Design review of the part built by this model. Coordinates are the model's own, in mm. A direction names the side the tool comes from. Give positions to 0.01 mm unless a question says otherwise; leave off trailing zeros. Write each loop counter-clockwise with the first axis right and the second up, starting at its lowest first coordinate (ties: lowest second). Pieces come first, ordered by that corner, then holes.
```python
from build123d import *

# Parameters (mm, degrees)
ESQUISSE1_R             = 25
ESQUISSE1_R_2           = 11.5
BOSS_EXTRU_1_DEPTH      = 8
ESQUISSE2_R             = 2.5
ENL_V_MAT_EXTRU_1_DEPTH = 37.249137921
ESQUISSE4_R             = 3.75
ENL_V_MAT_EXTRU_2_DEPTH = 5
ENL_V_START             = -14
ENL_V_MAT_EXTRU_7_DEPTH = 10
ESQUISSE10_R            = 4.25
ENL_V_MAT_EXTRU_5_DEPTH = 3.5
ESQUISSE12_R            = 4.25
ENL_V_MAT_EXTRU_6_DEPTH = 3.5


with BuildPart() as part:
    # Esquisse1 → Boss.-Extru.1 (new body)
    with BuildSketch(Plane.XY):
        Circle(ESQUISSE1_R)
        Circle(ESQUISSE1_R_2, mode=Mode.SUBTRACT)
    extrude(amount=BOSS_EXTRU_1_DEPTH)

    # Esquisse2 → Enlèv. mat.-Extru.1 (cut, through all)
    with BuildSketch(Plane.XY.offset(8)):
        with Locations((-14.713385832, 6.286197369)):
            Circle(ESQUISSE2_R)
        with Locations((6.28955657, 14.711950182)):
            Circle(ESQUISSE2_R)
        with Locations((14.713385832, -6.286197369)):
            Circle(ESQUISSE2_R)
        with Locations((-6.28955657, -14.711950182)):
            Circle(ESQUISSE2_R)
    extrude(amount=-ENL_V_MAT_EXTRU_1_DEPTH, mode=Mode.SUBTRACT)

    # Esquisse4 → Enlèv. mat.-Extru.2 (cut)
    with BuildSketch(Plane.XY.offset(8)):
        with Locations((-6.28955657, -14.711950182)):
            Circle(ESQUISSE4_R)
        with Locations((14.713385832, -6.286197369)):
            Circle(ESQUISSE4_R)
        with Locations((6.28955657, 14.711950182)):
            Circle(ESQUISSE4_R)
        with Locations((-14.713385832, 6.286197369)):
            Circle(ESQUISSE4_R)
    extrude(amount=-ENL_V_MAT_EXTRU_2_DEPTH, mode=Mode.SUBTRACT)

    # Esquisse13 → Enlèv. mat.-Extru.7 (cut)
    with BuildSketch(Plane(origin=(0, 0, 0), x_dir=(-0.9281017411356184, -0.3723266819622707, 0), z_dir=(-0.3723266819622707, 0.9281017411356184, 0)).offset(ENL_V_START)):
        Polygon((-2.5, 8), (2.5, 8), (0.5, 5.763932023), (-0.5, 5.763932023), align=None)
    enl_v_mat_extru_7 = extrude(amount=-ENL_V_MAT_EXTRU_7_DEPTH, mode=Mode.SUBTRACT)

    # Esquisse10 → Enlèv. mat.-Extru.5 (cut)
    with BuildSketch(Plane(origin=(0, 0, 0), x_dir=(-1, 0, 0), z_dir=(0, 0, -1))):
        with Locations((7.074206957, 17.633933082)):
            Circle(ESQUISSE10_R)
        with Locations((-7.074206957, -17.633933082)):
            Circle(ESQUISSE10_R)
    extrude(amount=-ENL_V_MAT_EXTRU_5_DEPTH, mode=Mode.SUBTRACT)

    # Esquisse12 → Enlèv. mat.-Extru.6 (cut)
    with BuildSketch(Plane.XY.offset(8)):
        with Locations((17.633933082, 7.074206957)):
            Circle(ESQUISSE12_R)
        with Locations((-17.633933082, -7.074206957)):
            Circle(ESQUISSE12_R)
    extrude(amount=-ENL_V_MAT_EXTRU_6_DEPTH, mode=Mode.SUBTRACT)

    # Symétrie1: Enlèv. mat.-Extru.7 across plane
    add(enl_v_mat_extru_7.mirror(Plane(origin=(0, 0, 0), x_dir=(0, 0, 1), z_dir=(-0.3723266819622707, 0.9281017411356184, 0))), mode=Mode.SUBTRACT)


solid = part.part
```
(1) Consider section C-C, the plane z = 1.5. Give the boundary of the cut face in (x, y), then the cut area to 3 significant figures.
Resolved:
outline: circle Ø50 at (0, 0); hole circle Ø5 at (-14.71, 6.29); hole circle Ø23 at (0, 0); hole circle Ø8.5 at (-7.07, 17.63); hole circle Ø5 at (-6.29, -14.71); hole circle Ø8.5 at (7.07, -17.63); hole circle Ø5 at (6.29, 14.71); hole circle Ø5 at (14.71, -6.29)
area: 1,360 mm2
(2) To check wall thickness, follow L1, parallel to Y at x = -8.5, z = 7.5; L2, parallel to Y at x = 4, z = 3.25; L3, parallel to X at y = 9.5, z = 6. State the ranges of each line that lie inside material, in increasing order.
Resolved:
L1: y = -23.51 to -17.74, -11.68 to -7.75, 7.75 to 15.67, 22.45 to 23.51
L2: y = -24.68 to -20.57, -14.7 to -10.78, 10.78 to 11.74, 17.68 to 24.68
L3: x = -23.12 to -16.65, -12.78 to -6.48, 6.48 to 14.14, 21.12 to 23.12
(3) Mouldability with a two-part tool opening along X and no side actions: class faces 4 (the face through (23.846, 7.509, 3.944)), 5 (the face through (-7, 18, 5.764)), 6 (the face through (11, -5, 8)) as pulls with the +X half, pulls with the -X half, needs draft (parallel to the pull), parting line crosses it, or undercut.
Resolved:
face 4: parting line crosses it
face 5: undercut
face 6: needs draft
(4) Tool access review of faces 1 (the face through (-12, 6, 3)), 2 (the face through (-7, 18, 3.5)), 3 (the face through (-16.697, 4.765, 1.521)): name each direction out of +Z, -Z, +X, -X, +Y, -Y from which nothing blocks a thin tool from reaching the whole face with its end or side.
Resolved:
face 1: +Z
face 2: -Z
face 3: +Z, -Z
(5) Clearance check with flat-ended pins moving along their axes: P1, Ø1.5, axis at y = -10, z = 4, coming from the +X side; P2, Ø8, axis at x = -14.71, y = 6.29, coming from the +Z side; P3, Ø1.4, axis at x = -7, y = 19, coming from the +Z side; P4, Ø4, axis at x = 8.5, y = -17.5, coming from the -Z side. State where each tip first meets the part, or that it passes through.
Resolved:
P1: stops at x = 23.23
P2: stops at z = 8
P3: stops at z = 6.63
P4: stops at z = 3.5
(6) Consider section A-A, the plane y = 0. Give the boundary of the cut face in (x, z), then the cut area to 3 significant figures.
Resolved:
outline: (-25, 0) - (-11.5, 0) - (-11.5, 8) - (-25, 8) - close; (11.5, 0) - (25, 0) - (25, 8) - (11.5, 8) - close
area: 216 mm2
(7) Consider section D-D, the plane y = 20. Give the boundary of the cut face in (x, z), then the cut area to 3 significant figures.
Resolved:
outline: (-15, 0) - (-10.6, 0) - (-10.6, 3.5) - (-3.54, 3.5) - (-3.54, 0) - (15, 0) - (15, 8) - (-5.33, 8) - (-7.48, 5.76) - (-8.56, 5.76) - (-10.72, 8) - (-15, 8) - close
area: 208 mm2
